Autodesk Inventor part; units mm, degrees
ref_plane "YZ Plane" through (0, 0, 0) normal (1, 0, 0) x (0, 1, 0)
ref_plane "XZ Plane" through (0, 0, 0) normal (0, 1, 0) x (-1, 0, 0)
ref_plane "XY Plane" through (0, 0, 0) normal (0, 0, 1) x (1, 0, 0)
sketch "Sketch1" plane through (0, 0, 0) normal (0, 0, 1) x (1, 0, 0)
  arc A0 (8.3864, -11.505) -> (3.6136, -11.505) centre (6, -6) ccw construction
  line L0 (-28.75, -36) -> (40.75, -36)
  line L1 (40.75, -36) -> (40.75, 24)
  line L2 (40.75, 24) -> (-28.75, 24)
  line L3 (-28.75, 24) -> (-28.75, -36)
  line L4 (-28.75, -36) -> (40.75, 24) construction
  line L5 (40.75, -36) -> (-28.75, 24) construction
  line L6 (12, 0) -> (0, 0)
  line L7 (0, 0) -> (0, -23)
  line L8 (0, -23) -> (12, -23)
  line L9 (12, -23) -> (12, 0)
  line L10 (-0.1, -23.1) -> (12.1, -23.1)
  line L11 (12.1, -23.1) -> (12.1, 0.1)
  line L12 (12.1, 0.1) -> (-0.1, 0.1)
  line L13 (-0.1, 0.1) -> (-0.1, -23.1)
  line L14 (-28.75, -6) -> (40.75, -6) construction
  line L15 (6, -36) -> (6, 24) construction
  line L16 (-28.75, -18) -> (-25.75, -18)
  line L17 (-25.75, -18) -> (-25.75, 6)
  line L18 (-25.75, 6) -> (-28.75, 6)
  line L19 (-28.75, 6) -> (-28.75, -18)
  line L20 (40.75, -18) -> (37.75, -18)
  line L21 (37.75, -18) -> (37.75, 6)
  line L22 (37.75, 6) -> (40.75, 6)
  line L23 (40.75, 6) -> (40.75, -18)
  arc A1 (6.5, -26.804) -> (5.5, -26.804) centre (6, -25.55) ccw construction
  arc A2 (5.5, 3.804) -> (6.5, 3.804) centre (6, 2.55) ccw construction
  circle A3 centre (6, -25.55) radius 1.35
  circle A4 centre (6, 2.55) radius 1.35
  dimension "d0" = 69.5
  dimension "d1" = 60
  dimension "d2" = 0.1
  dimension "d3" = 0.1
  dimension "d4" = 0.1
  dimension "d5" = 0.1
  dimension "d6" = 12
  dimension "d7" = 12
  dimension "d8" = 3
extrude "Extrusion1" add sketch "Sketch1" along normal blind 3 contours L3 L16 L17 L18 L2 L1 L22 L21 L20 L0
sketch "Sketch2" plane through (0, 0, 0) normal (0, 0, -1) x (-1, 0, 0)
  circle A0 centre (15.85, 19) radius 1.8
  circle A1 centre (-27.85, 19) radius 1.8
  circle A2 centre (-27.85, -31) radius 1.8
  circle A3 centre (15.85, -31) radius 1.8
  point P0 (0, 0)
extrude "Extrusion2" cut sketch "Sketch2" against normal blind 7.7625
sketch "Sketch3" plane through (0, 0, 3) normal (0, 0, 1) x (1, 0, 0)
  line L0 (-14.9463, -12.3199) -> (-9.9463, -20.9801) construction
  line L1 (-17.5444, -13.8199) -> (-12.5444, -22.4801) construction
  line L2 (-12.5444, -22.4801) -> (-9.9463, -20.9801) construction
  line L3 (-17.5444, -13.8199) -> (-14.9463, -12.3199) construction
  line L4 (29.5444, -13.8199) -> (26.9463, -12.3199) construction
  line L5 (24.5444, -22.4801) -> (21.9463, -20.9801) construction
  line L6 (21.9463, -20.9801) -> (26.9463, -12.3199) construction
  line L7 (24.5444, -22.4801) -> (29.5444, -13.8199) construction
  line L8 (11, 15.3) -> (1, 15.3) construction
  line L9 (11, 18.3) -> (1, 18.3) construction
  line L10 (11, 18.3) -> (11, 15.3) construction
  line L11 (1, 18.3) -> (1, 15.3) construction
  line L12 (26.9646, -12.3882) -> (29.4761, -13.8382)
  line L13 (29.4761, -13.8382) -> (24.5261, -22.4118)
  line L14 (24.5261, -22.4118) -> (22.0146, -20.9618)
  line L15 (22.0146, -20.9618) -> (26.9646, -12.3882)
  line L16 (-10.0146, -20.9618) -> (-14.9646, -12.3882)
  line L17 (-14.9646, -12.3882) -> (-17.4761, -13.8382)
  line L18 (-17.4761, -13.8382) -> (-12.5261, -22.4118)
  line L19 (-12.5261, -22.4118) -> (-10.0146, -20.9618)
  line L20 (1.05, 15.35) -> (10.95, 15.35)
  line L21 (10.95, 15.35) -> (10.95, 18.25)
  line L22 (10.95, 18.25) -> (1.05, 18.25)
  line L23 (1.05, 18.25) -> (1.05, 15.35)
  point P0 (0, 0)
  dimension "d13" = 0.05
  dimension "d14" = 0.05
  dimension "d15" = 0.05
extrude "Extrusion3" cut sketch "Sketch3" against normal blind 10
properties part number "Camera pan base"
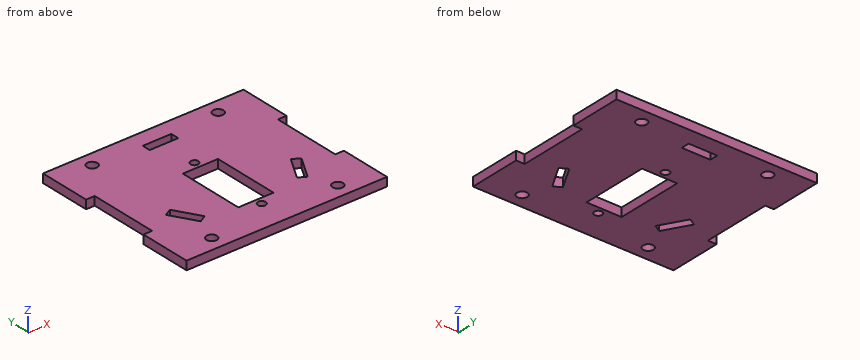
Can you work these out from the model? Positions are in its coordinate system, mm. Coordinates: 2 decimals unless noted, no trailing zeros. Order: outer loops, then holes, each group sorted by start corner. A loop starts at its lowest first (then second) coordinate and runs counter-clockwise, first axis right, second up. Notation, with made-up numbers: (87, 37.25) - (99, 37.25) arc R29 cw to (99, 69.25) - close; hole circle Ø8 at (34.25, 48). An arc over 180 degrees is marked (long way). Answer as a JSON object with one key per item and string values. Group by question number.
Q1. I need wall thicknesses on line 1 (X direction, y = -6, z = 1.8); line 2 (Y direction, x = 0.5, z = 0.5); line 3 (Y direction, x = 6, z = 1.6). Which ranges of each line are inside material? Lowest first, please. Write a range as from..to.
Q2. Imagine slicing it at A-A (y = -31). Please give me the cut outline in (x, z), and give its area (3 significant figures).
Q3. Imagine slicing it at B-B (z = 1). Give the number of separate pieces and of enclosed holes in the cut face, and give its area (3 significant figures).
Q4. Will these pins go through, and if not, where does the flat tip stop? P1, Ø1.5, axis at y = -7, z = 2, coming from the -X side; P2, Ø1.5, axis at y = -1.5, z = 2, coming from the +X side.
Q5. Imagine slicing it at C-C (x = 6). Please give me the cut outline in (y, z).
Q6. Imagine slicing it at D-D (x = -15.85). Please give me the cut outline in (y, z).
Determined:
{
 "1": {"line 1": "x = -25.75..-0.1, 12.1..37.75", "line 2": "y = -36..-23.1, 0.1..24", "line 3": "y = -36..-26.9, -24.2..-23.1, 0.1..1.2, 3.9..15.35, 18.25..24"},
 "2": {"outline": "(-28.75, 0) - (-17.65, 0) - (-17.65, 3) - (-28.75, 3) - close; (-14.05, 0) - (26.05, 0) - (26.05, 3) - (-14.05, 3) - close; (29.65, 0) - (40.75, 0) - (40.75, 3) - (29.65, 3) - close", "area": "187 mm2"},
 "3": {"separate pieces": "1", "enclosed holes": "10", "area": "3,600 mm2"},
 "4": {"P1": "stops at x = -25.75", "P2": "stops at x = 37.75"},
 "5": {"outline": "(-36, 0) - (-26.9, 0) - (-26.9, 3) - (-36, 3) - close; (-24.2, 0) - (-23.1, 0) - (-23.1, 3) - (-24.2, 3) - close; (0.1, 0) - (1.2, 0) - (1.2, 3) - (0.1, 3) - close; (3.9, 0) - (15.35, 0) - (15.35, 3) - (3.9, 3) - close; (18.25, 0) - (24, 0) - (24, 3) - (18.25, 3) - close"},
 "6": {"outline": "(-36, 0) - (-32.8, 0) - (-32.8, 3) - (-36, 3) - close; (-29.2, 0) - (-16.65, 0) - (-16.65, 3) - (-29.2, 3) - close; (-12.9, 0) - (17.2, 0) - (17.2, 3) - (-12.9, 3) - close; (20.8, 0) - (24, 0) - (24, 3) - (20.8, 3) - close"}
}
